```python
from build123d import *

# Parameters (mm, degrees)
BOSS_EXTRUDE1_DEPTH               = 1.3
BOSS_EXTRUDE2_DEPTH               = 12
CUT_TO_REMOVE_BOT_SOLE_DEPTH      = 234.592504803
CUT_TO_REMOVE_BOT_SOLE_DEPTH_BACK = 234.592504803
CUT_EXTRUDE4_REACH                = 167.31
SKETCH7_W                         = 18.70749212
SKETCH7_H                         = 9
SKETCH7_W_2                       = 17.851063772


with BuildPart() as part:
    # Sketch2 → Boss-Extrude1 (new body)
    with BuildSketch(Plane(origin=(0, 0, 0), x_dir=(1, 0, 0), z_dir=(0, 1, 0))):
        with BuildLine():
            add(Edge.make_bspline(
                [(23.05, 127), (22.943163576, 126.902857828), (6.620867571, 120.021081895), (0.931086245, 101.488970464), (0.324008086, 88.719210316), (3.825949637, 76.00589269), (8.107522159, 63.165811678), (14.622542207, 50.857319444), (20.477621735, 37.804703348), (28.027386546, 24.819252915), (38.054220669, 12.174080363), (50.087048562, -0.413905353), (63.515875121, -12.714926203), (76.995002025, -24.637109723), (87.753725412, -37.676814115), (96.95133677, -50.066381), (102.490643182, -63.337711531), (106.915198332, -76.285665463), (112.18840739, -88.815145737), (116.555805718, -101.829881852), (122.760488068, -115.656378348), (136.34325775, -130.188055829), (151.998790453, -139.029236195), (161.96, -136.1)],
                knots=[0, 0, 0, 0, 0.090945349, 0.12664197, 0.163655193, 0.201591738, 0.240816764, 0.281850131, 0.322917617, 0.365825557, 0.412648122, 0.463551179, 0.517804141, 0.571801955, 0.620389186, 0.665335117, 0.705885892, 0.745281612, 0.78501862, 0.824424381, 0.865568121, 0.915423297, 1, 1, 1, 1], degree=3))
            add(Edge.make_bspline(
                [(161.96, -136.1), (172.431616467, -132.923660625), (186.600337708, -121.715263252), (189.399120136, -101.609128058), (188.081273674, -88.738164313), (184.889467755, -75.876127028), (179.456656008, -63.289286222), (173.0414801, -50.841874911), (166.79981093, -38.270821821), (161.60365795, -25.396077846), (156.248349303, -12.794060465), (151.450238349, -0.096351247), (147.526781794, 12.914664382), (141.825873335, 25.26402088), (137.37019782, 38.220879174), (131.875071866, 50.794972902), (126.706198444, 64.316783566), (117.282300149, 76.451578571), (103.420435284, 93.759455253), (86.842392664, 113.310643183), (58.200495652, 131.153143927), (35.386261, 132.287626366), (23.05, 127)],
                knots=[0, 0, 0, 0, 0.095093522, 0.131398848, 0.167295759, 0.204174646, 0.242856644, 0.282808561, 0.322537216, 0.361360107, 0.400063589, 0.438231587, 0.476003009, 0.514706491, 0.552943744, 0.591625742, 0.630784901, 0.674461238, 0.720301597, 0.818758385, 0.889157941, 1, 1, 1, 1], degree=3))
        make_face()
    extrude(amount=-BOSS_EXTRUDE1_DEPTH)

    # Sketch3 → Boss-Extrude2 (add)
    with BuildSketch(Plane(origin=(0, 0, 0), x_dir=(1, 0, 0), z_dir=(0, 1, 0))):
        with BuildLine():
            add(Edge.make_bspline(
                [(23.05, 127), (22.943163576, 126.902857828), (6.620867571, 120.021081895), (0.931086245, 101.488970464), (0.324008086, 88.719210316), (3.825949637, 76.00589269), (8.107522159, 63.165811678), (14.622542207, 50.857319444), (18.754484417, 41.646060206), (21.253091273, 36.855386406), (21.582029576, 36.236743436)],
                knots=[0, 0, 0, 0, 0.090945349, 0.12664197, 0.163655193, 0.201591738, 0.240816764, 0.281850131, 0.322917617, 0.329035738, 0.329035738, 0.329035738, 0.329035738], degree=3))
            Line((21.582029576, 36.236743436), (111.276939854, 83.928373203))
            add(Edge.make_bspline(
                [(111.276939854, 83.928373203), (109.94087902, 85.589385686), (101.272885125, 96.292152129), (86.842392664, 113.310643183), (58.200495652, 131.153143927), (35.386261, 132.287626366), (23.05, 127)],
                knots=[0.702273444, 0.702273444, 0.702273444, 0.702273444, 0.720301597, 0.818758385, 0.889157941, 1, 1, 1, 1], degree=3))
        make_face()
        Polygon((23.877677337, 71.434462523), (11.671416705, 94.391099938), (60.233534312, 120.212035891), (72.439794944, 97.255398476), align=None, mode=Mode.SUBTRACT)
    extrude(amount=BOSS_EXTRUDE2_DEPTH)

    # Sketch6 → Cut to remove bot sole (cut, two sides: drawn at the far end of the back side and taken through both)
    with BuildSketch(Plane(origin=(0, 0, 0), x_dir=(1, 0, 0), z_dir=(0, 1, 0)).offset(-CUT_TO_REMOVE_BOT_SOLE_DEPTH_BACK)):
        with BuildLine():
            Line((111.276939854, 83.928373203), (21.582029576, 36.236743436))
            add(Edge.make_bspline(
                [(21.582029576, 36.236743436), (23.560019233, 32.51668594), (28.463593854, 24.269137433), (38.054220669, 12.174080363), (50.087048562, -0.413905353), (63.515875121, -12.714926203), (76.995002025, -24.637109723), (87.753725412, -37.676814115), (96.95133677, -50.066381), (102.490643182, -63.337711531), (106.915198332, -76.285665463), (112.18840739, -88.815145737), (116.555805718, -101.829881852), (122.760488068, -115.656378348), (136.34325775, -130.188055829), (151.998790453, -139.029236195), (161.96, -136.1)],
                knots=[0.329035738, 0.329035738, 0.329035738, 0.329035738, 0.365825557, 0.412648122, 0.463551179, 0.517804141, 0.571801955, 0.620389186, 0.665335117, 0.705885892, 0.745281612, 0.78501862, 0.824424381, 0.865568121, 0.915423297, 1, 1, 1, 1], degree=3))
            add(Edge.make_bspline(
                [(161.96, -136.1), (172.431616467, -132.923660625), (186.600337708, -121.715263252), (189.399120136, -101.609128058), (188.081273674, -88.738164313), (184.889467755, -75.876127028), (179.456656008, -63.289286222), (173.0414801, -50.841874911), (166.79981093, -38.270821821), (161.60365795, -25.396077846), (156.248349303, -12.794060465), (151.450238349, -0.096351247), (147.526781794, 12.914664382), (141.825873335, 25.26402088), (137.37019782, 38.220879174), (131.875071866, 50.794972902), (126.706198444, 64.316783566), (118.602637041, 74.751431029), (113.338093865, 81.365913132), (111.276939854, 83.928373203)],
                knots=[0, 0, 0, 0, 0.095093522, 0.131398848, 0.167295759, 0.204174646, 0.242856644, 0.282808561, 0.322537216, 0.361360107, 0.400063589, 0.438231587, 0.476003009, 0.514706491, 0.552943744, 0.591625742, 0.630784901, 0.674461238, 0.702273444, 0.702273444, 0.702273444, 0.702273444], degree=3))
        make_face()
    extrude(amount=CUT_TO_REMOVE_BOT_SOLE_DEPTH + CUT_TO_REMOVE_BOT_SOLE_DEPTH_BACK, mode=Mode.SUBTRACT)

    # Sketch7 → Cut-Extrude4 (cut, up to next)
    with BuildSketch(Plane(origin=(-10.264055011, 0, -19.3038799), x_dir=(0.8829475928589329, 0, -0.46947156278587965), z_dir=(0.46947156278587965, 0, 0.8829475928589329)), mode=Mode.PRIVATE) as cut_extrude4_sk1:
        with Locations((63.972932545, 4.5)):
            Rectangle(SKETCH7_W, SKETCH7_H)
    cut_extrude4_tool1 = extrude(cut_extrude4_sk1.sketch, amount=-CUT_EXTRUDE4_REACH, mode=Mode.PRIVATE) & part.part
    # Sketch7 → Cut-Extrude4 (cut, up to next)
    with BuildSketch(Plane(origin=(-10.264055011, 0, -19.3038799), x_dir=(0.8829475928589329, 0, -0.46947156278587965), z_dir=(0.46947156278587965, 0, 0.8829475928589329)), mode=Mode.PRIVATE) as cut_extrude4_sk2:
        with Locations((100.693654599, 4.5)):
            Rectangle(SKETCH7_W_2, SKETCH7_H)
    cut_extrude4_tool2 = extrude(cut_extrude4_sk2.sketch, amount=-CUT_EXTRUDE4_REACH, mode=Mode.PRIVATE) & part.part
    add(cut_extrude4_tool1.solids().sort_by_distance((46.220692, 4.5, -49.337353))[0], mode=Mode.SUBTRACT)
    add(cut_extrude4_tool2.solids().sort_by_distance((78.643165, 4.5, -66.576687))[0], mode=Mode.SUBTRACT)


solid = part.part
```
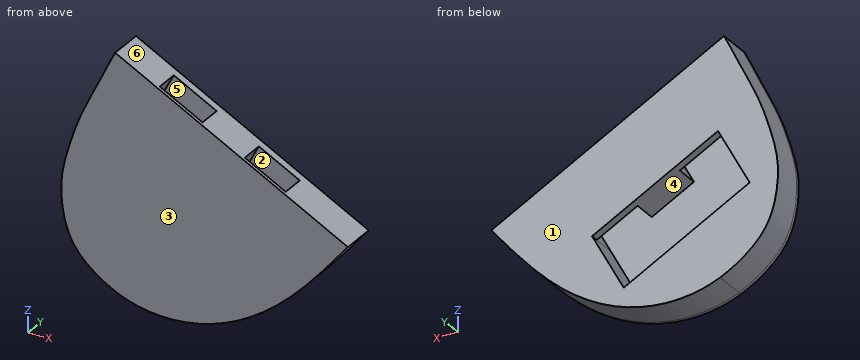
Can you work these out from the model? Positions are in its coordinate system, mm. Face numbers are marked on the shaded views. A direction names the side the tool comes from. Give positions to 0.01 mm unless a question says otherwise; leave off trailing zeros. Answer in a Markdown table with one row per item.
1. For pin 1 Ø12 at (x, z) = (53.5, -104.5) entering from +Y; pin 2 Ø1.5 at (y, z) = (2, -119) entering from +X; pin 3 Ø2 at (x, y) = (54.5, 9) entering from -Z, each with a flat end and sliding along its axis, tell me the tip position at first contact or that it passes through.
Taken from the geometry:
| item | result |
|---|---|
| pin 1 | stops at y = 0 |
| pin 2 | stops at x = 78.04 |
| pin 3 | stops at z = -129.41 |
2. Which directions (+Z, -Z, +X, -X, +Y, -Y) give clear straight access to the entire face, cutting with the end or side of a thin tool? Please do the marked faces 5 and 6.
Taken from the geometry:
| item | result |
|---|---|
| face 5 | none |
| face 6 | +Z, +X, +Y, -Y |
3. If I drill on line 1 along Y through (x, z) = (38, -53.5); line 2 along X through (y, z) = (8, -83.5); line 3 along X through (y, z) = (5, -74), over which ranges is the centre line in solid material (lowest first)?
Taken from the geometry:
| item | result |
|---|---|
| line 1 | y = -1.3 to 0, 9 to 12 |
| line 2 | x = 1.91 to 17.46, 46.57 to 59.54, 79.75 to 110.47 |
| line 3 | x = 4.57 to 22.51, 43.7 to 64.59, 84.8 to 92.6 |
4. Thinking about a two-plate mould opening in Y: for the marked faces 1, 2, 3 and 4, which applies, released by +Y, released by -Y, zero draft, split by the parting line, or undercut?
Taken from the geometry:
| item | result |
|---|---|
| face 1 | released by +Y |
| face 2 | undercut |
| face 3 | released by -Y |
| face 4 | zero draft |
